Here's the drawing with two shaded views (mm, measured from the low corner). I have some questions. Round coordinates to 2 decimals unless told otherwise and drop trailing zeros. Order: outer loops, then holes, each group sorted by start corner. A loop starts at its lowest first (then second) coordinate and runs counter-clockwise, first axis right, second up.
Q1. If we section it at A-A (x = 17.5): Please give me the cut outline in (y, z), plus the area to 3 significant figures.
Q2. If I drill on line 1 (X direction, y = 77.5, z = 19); line 2 (X direction, y = 68, z = 23); line 3 (Y direction, x = 17, z = 4), over which ranges is the centre line in solid material (lowest first)?
Q3. If we section it at B-B (y = 50): Please give me the cut outline in (x, z).
Q4. If we section it at D-D (y = 21): Please give me the cut outline in (x, z), plus the area to 3 significant figures.
Q5. If we section it at C-C (z = 10.5): Please give me the cut outline in (x, y).
Q6. Will these pins go through, and if not, where does the flat tip stop? P1, Ø2, axis at x = 13, y = 21.5, coming from the +Z side; P2, Ø8, axis at x = 12, y = 33.5, coming from the +Z side; P3, Ø7.5, axis at x = 17.5, y = 50, coming from the +Z side.
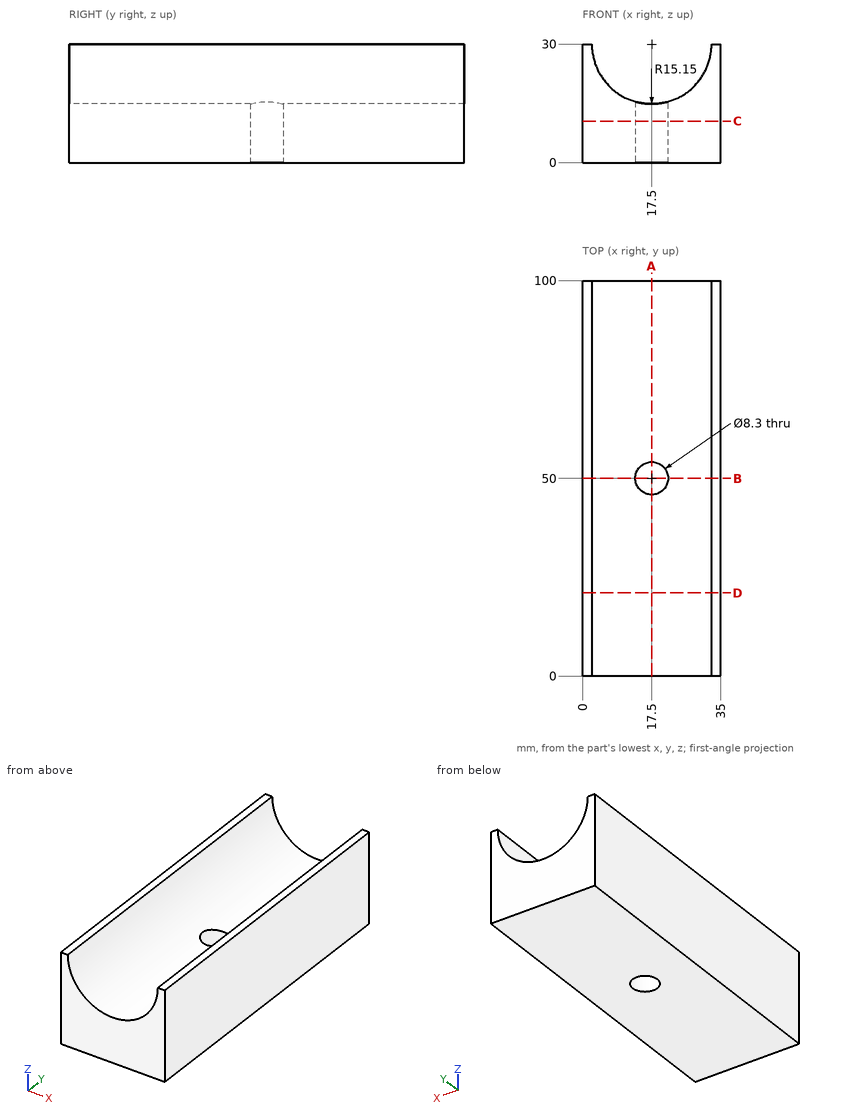
Solution:
1. outline: (0, 0) - (45.85, 0) - (45.85, 14.85) - (0, 14.85) - close; (54.15, 0) - (100, 0) - (100, 14.85) - (54.15, 14.85) - close
1. area: 1,360 mm2
2. line 1: x = 0 to 7.08, 27.92 to 35
2. line 2: x = 0 to 4.06, 30.94 to 35
2. line 3: y = 0 to 45.88, 54.12 to 100
3. outline: (0, 0) - (13.35, 0) - (13.35, 15.43) arc R15.15 cw to (2.35, 30) - (0, 30) - close; (21.65, 0) - (35, 0) - (35, 30) - (32.65, 30) arc R15.15 cw to (21.65, 15.43) - close
4. outline: (0, 0) - (35, 0) - (35, 30) - (32.65, 30) arc R15.15 cw to (2.35, 30) - (0, 30) - close
4. area: 689 mm2
5. outline: (0, 0) - (35, 0) - (35, 100) - (0, 100) - close; hole circle Ø8.3 at (17.5, 50)
6. P1: stops at z = 15.88
6. P2: stops at z = 18.2
6. P3: passes through
